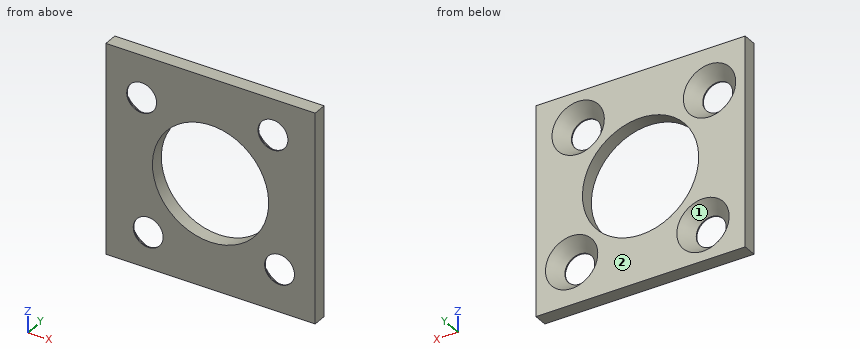
from build123d import *

# Parameters (mm, degrees)
SKETCH1_W                                     = 22.86
SKETCH1_H                                     = 22.86
SKETCH1_R                                     = 6.35
BOSS_EXTRUDE1_DEPTH                           = 1.524
CSK_FOR_4_FLAT_HEAD_MACHINE_SCREW1_AT_2_COUNT = 2
CSK_FOR_4_FLAT_HEAD_MACHINE_SCREW1_AT_2_PITCH = 14.368409794
CSK_FOR_4_FLAT_HEAD_MACHINE_SCREW1_AT_3_COUNT = 2
CSK_FOR_4_FLAT_HEAD_MACHINE_SCREW1_AT_3_PITCH = 20.32
CSK_FOR_4_FLAT_HEAD_MACHINE_SCREW1_AT_4_COUNT = 2
CSK_FOR_4_FLAT_HEAD_MACHINE_SCREW1_AT_4_PITCH = 14.368409794


with BuildPart() as part:
    # Sketch1 → Boss-Extrude1 (new body)
    with BuildSketch(Plane(origin=(0, 0, 0), x_dir=(1, 0, 0), z_dir=(0, 1, 0))):
        with Locations((-11.43, 11.43)):
            Rectangle(SKETCH1_W, SKETCH1_H)
        with Locations(Location((-11.43, 11.43, 0), (0, 0, 90))):
            Circle(SKETCH1_R, mode=Mode.SUBTRACT)
    extrude(amount=BOSS_EXTRUDE1_DEPTH)

    # Sketch3 → CSK for #4 Flat Head Machine Screw1 (revolve, cut)
    with BuildSketch(Plane(origin=(-3.897724655, 1.524, -18.248388969), x_dir=(0, 0, 1), z_dir=(1, 0, 0))):
        Polygon((0, 0), (0, 1.524), (1.63195, 1.524), (1.63195, 1.409834001), (2.8575, 0), align=None)
    csk_for_4_flat_head_machine_screw1 = revolve(axis=Axis((-3.897724655, 7.874, -18.248388969), (0, -1, 0)), mode=Mode.SUBTRACT)

    # CSK for #4 Flat Head Machine Screw1 at 2: CSK for #4 Flat Head Machine Screw1 ×2
    with Locations(*[Vector(-0.049684438764001596, 0, 0.99876496561739) * (i * CSK_FOR_4_FLAT_HEAD_MACHINE_SCREW1_AT_2_PITCH) for i in range(1, CSK_FOR_4_FLAT_HEAD_MACHINE_SCREW1_AT_2_COUNT)]):
        add(csk_for_4_flat_head_machine_screw1, mode=Mode.SUBTRACT)

    # CSK for #4 Flat Head Machine Screw1 at 3: CSK for #4 Flat Head Machine Screw1 ×2
    with Locations(*[Vector(-0.7413656835690785, 0, 0.6711012764301324) * (i * CSK_FOR_4_FLAT_HEAD_MACHINE_SCREW1_AT_3_PITCH) for i in range(1, CSK_FOR_4_FLAT_HEAD_MACHINE_SCREW1_AT_3_COUNT)]):
        add(csk_for_4_flat_head_machine_screw1, mode=Mode.SUBTRACT)

    # CSK for #4 Flat Head Machine Screw1 at 4: CSK for #4 Flat Head Machine Screw1 ×2
    with Locations(*[Vector(-0.99876496561739, 0, -0.04968443876400101) * (i * CSK_FOR_4_FLAT_HEAD_MACHINE_SCREW1_AT_4_PITCH) for i in range(1, CSK_FOR_4_FLAT_HEAD_MACHINE_SCREW1_AT_4_COUNT)]):
        add(csk_for_4_flat_head_machine_screw1, mode=Mode.SUBTRACT)


solid = part.part
Build history of the part. All positions in model axes, mm. Face numbers are marked on the shaded views. Coordinates: 2 decimals unless noted, no trailing zeros. Order: outer loops, then holes, each group sorted by start corner. A loop starts at its lowest first (then second) coordinate and runs counter-clockwise, first axis right, second up. Notation, with made-up numbers: (16.5, 49) - (45.5, 49) arc R16 cw to (45.5, 54) - close; hole circle Ø7 at (8.25, 22.25). An arc over 180 degrees is marked (long way). Write each question's results on one line, items separated by ' | '. Start each with the question number.
Item 1: Mould opens along X. For the marked faces 1 and 2 say: released by +X, released by -X, zero draft, split by the parting line, or undercut.
Item 2: Band-saw the part on A-A on x = -11.43. Write the cut outline in (y, z).
Item 3: Band-saw the part on C-C on y = 0.4. Write the cut outline in (x, z).
Item 4: Band-saw the part on B-B on z = -11.43. Write the cut outline in (x, y).
Item 5: Wall check: probe 1 along X at (y, z) = (0.35, -3.5) (3 decimals); probe 2 along X at (y, z) = (0.5, -5); probe 3 along Z at (x, y) = (-2.5, 1.4). Give the ranges that are in metal, low to high. Write a range as [from, to].
Numbers:
1) face 1: undercut | face 2: zero draft
2) outline: (0, -22.86) - (1.52, -22.86) - (1.52, -17.78) - (0, -17.78) - close; (0, -5.08) - (1.52, -5.08) - (1.52, 0) - (0, 0) - close
3) outline: (-22.86, -22.86) - (0, -22.86) - (0, 0) - (-22.86, 0) - close; hole circle Ø3.76 at (-18.96, -4.61); hole circle Ø3.76 at (-18.25, -18.96); hole circle Ø12.7 at (-11.43, -11.43); hole circle Ø3.76 at (-4.61, -3.9); hole circle Ø3.76 at (-3.9, -18.25)
4) outline: (-22.86, 0) - (-17.78, 0) - (-17.78, 1.52) - (-22.86, 1.52) - close; (-5.08, 0) - (0, 0) - (0, 1.52) - (-5.08, 1.52) - close
5) probe 1: [-22.86, -20.425], [-17.5, -6.405], [-2.818, 0] | probe 2: [-22.86, -20.89], [-17.03, -6.24], [-2.98, 0] | probe 3: [-22.86, -20.62], [-15.88, -5.66], [-2.14, 0]
